Could you check a few things on this drawing? It's one solid part, dimensions in mm from its lowest x, y, z. A direction names the side the tool comes from. Round coordinates to 2 decimals unless told otherwise and drop trailing zeros. Write each loop counter-clockwise with the first axis right and the second up, starting at its lowest first coordinate (ties: lowest second). Pieces come first, ordered by that corner, then holes. Notation, with made-up numbers: (47.25, 82.5) -> (92.25, 82.5) arc R19 cw to (92.25, 118.5) -> close; hole circle Ø8 at (61.5, 57.25). An arc over 180 degrees is marked (long way). Answer in a Markdown table with one row per item.
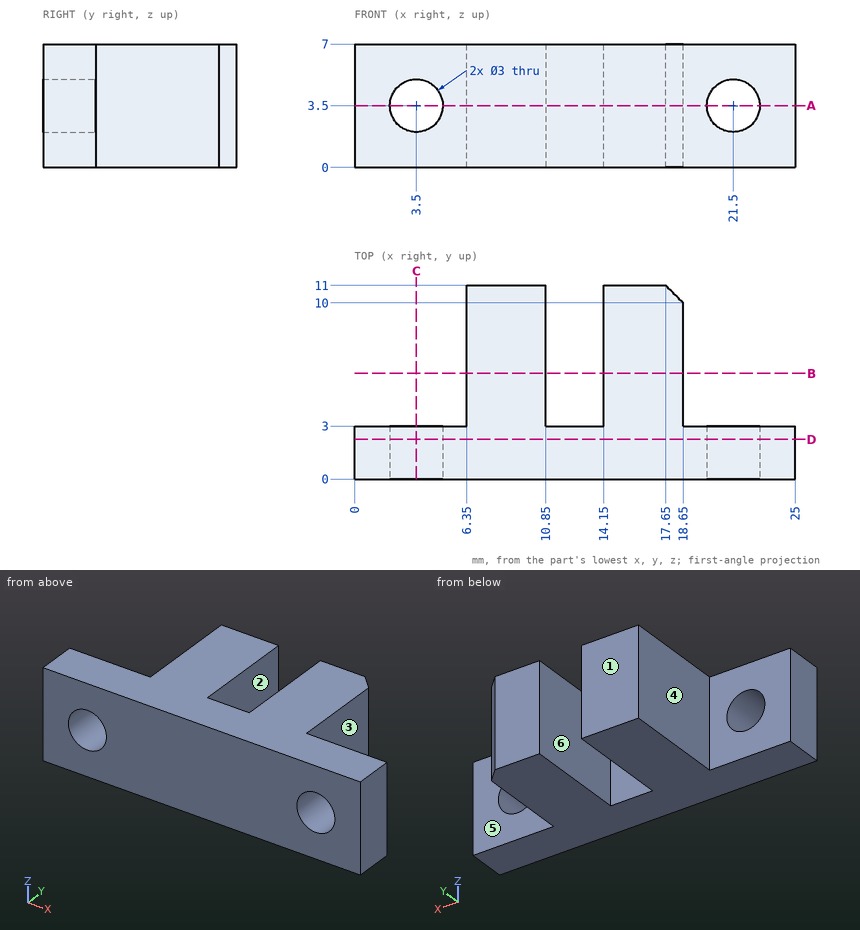
1) Imagine slicing it at B-B, the plane y = 6. Please give me the cut outline in (x, z).
Findings:
| item | result |
|---|---|
| outline | (6.35, 0) -> (10.85, 0) -> (10.85, 7) -> (6.35, 7) -> close; (14.15, 0) -> (18.65, 0) -> (18.65, 7) -> (14.15, 7) -> close |
2) Imagine slicing it at A-A, the plane z = 3.5. Please give me the cut outline in (x, y).
Findings:
| item | result |
|---|---|
| outline | (0, 0) -> (2, 0) -> (2, 3) -> (0, 3) -> close; (5, 0) -> (20, 0) -> (20, 3) -> (18.65, 3) -> (18.65, 10) -> (17.65, 11) -> (14.15, 11) -> (14.15, 3) -> (10.85, 3) -> (10.85, 11) -> (6.35, 11) -> (6.35, 3) -> (5, 3) -> close; (23, 0) -> (25, 0) -> (25, 3) -> (23, 3) -> close |
3) For pin 1 (1.9 mm diameter, centred on x = 2, z = 3, fed in from +Y); pin 2 (3.5 mm diameter, centred on y = 5.5, z = 4.5, fed in from +X); pin 3 (3.5 mm diameter, centred on y = 7.5, z = 2.5, fed in from -X), each with a flat end and sliding along its axis, tell me the tip position at first contact or that it passes through.
Findings:
| item | result |
|---|---|
| pin 1 | stops at y = 3 |
| pin 2 | stops at x = 18.65 |
| pin 3 | stops at x = 6.35 |
4) Please list where these lines run through material, in increasing order: line 1 (X direction, y = 2.3, z = 3.5); line 2 (Z direction, x = 3.5, y = 2.1); line 3 (X direction, y = 4.25, z = 2.25).
Findings:
| item | result |
|---|---|
| line 1 | x = 0 to 2, 5 to 20, 23 to 25 |
| line 2 | z = 0 to 2, 5 to 7 |
| line 3 | x = 6.35 to 10.85, 14.15 to 18.65 |
5) Thinking about a two-plate mould opening in X: for the marked faces 1, 2 and 3, which applies, +X half, -X half, draft (parallel to the pull), parting line (faces both ways), or undercut?
Findings:
| item | result |
|---|---|
| face 1 | draft |
| face 2 | undercut |
| face 3 | +X half |
6) For the marked faces 4, 5 and 6, which set-ups out of +Z, -Z, +X, -X, +Y, -Y let a thin tool reach every point of the face, with its end or its side?
Findings:
| item | result |
|---|---|
| face 4 | +Z, -Z, -X, +Y |
| face 5 | +Z, -Z, +X, +Y |
| face 6 | +Z, -Z, +Y |
7) Imagine slicing it at D-D, the plane y = 2.25. Please give me the cut outline in (x, z), plus the area to 3 significant figures.
Findings:
| item | result |
|---|---|
| outline | (0, 0) -> (25, 0) -> (25, 7) -> (0, 7) -> close; hole circle Ø3 at (3.5, 3.5); hole circle Ø3 at (21.5, 3.5) |
| area | 161 mm^2 |
8) Imagine slicing it at C-C, the plane x = 3.5. Please give me the cut outline in (y, z).
Findings:
| item | result |
|---|---|
| outline | (0, 0) -> (3, 0) -> (3, 2) -> (0, 2) -> close; (0, 5) -> (3, 5) -> (3, 7) -> (0, 7) -> close |
